Build history of the part. All positions in model axes, mm. Face numbers are marked on the shaded views. A direction names the side the tool comes from. Give positions to 0.01 mm unless a question says otherwise; leave off trailing zeros. Order: outer loops, then holes, each group sorted by start corner. A loop starts at its lowest first (then second) coordinate and runs counter-clockwise, first axis right, second up. Notation, with made-up numbers: (-7, 18.25) -> (50, 18.25) arc R27 ccw to (50, 57.25) -> close; hole circle Ø5 at (54, 2). An arc over 180 degrees is marked (long way). One line per item, written item: value. Start each with the question number.
(1) Saw through at B-B on z = -14.5. Give the cut face in (x, y), plus the area to 3 significant figures.
(2) Pin check, flat tips, straight feed: pin 1 (5 mm diameter, centred on x = 24, z = -0.5, fed in from +Y); pin 2 (1.6 mm diameter, centred on y = 0.5, z = 5, fed in from -X). Stop position of each tip, or through.
(3) Which spindle directions (+Z, -Z, +X, -X, +Y, -Y) get a long thin tool onto all of the face, cutting with end or side? Do the marked faces 5 and 6. Say none if no direction does.
(4) Saw through at A-A on x = -20. Give the cut face in (y, z), plus the area to 3 significant figures.
(5) Saw through at C-C on y = 3.25. Give the cut face in (x, z), plus the area to 3 significant figures.
(6) Probe line 1 (Z direction, x = 10.5, y = 4.5); line 2 (Z direction, x = 14, y = 4.25); line 3 (Z direction, x = -19, y = 6.75). List the from-to ranges inside material, lowest first.
(7) Saw through at D-D on x = -10.5. Give the cut face in (y, z).
(8) Two-plate mould, pull along X, no slides. Class the marked faces 1, 2, 3 and 4: +X half, -X half, draft (parallel to the pull), parting line (faces both ways), or undercut.
Autodesk Inventor part; units mm, degrees
ref_plane "YZ Plane" through (0, 0, 0) normal (1, 0, 0) x (0, 1, 0)
ref_plane "XZ Plane" through (0, 0, 0) normal (0, 1, 0) x (-1, 0, 0)
ref_plane "XY Plane" through (0, 0, 0) normal (0, 0, 1) x (1, 0, 0)
sketch "Sketch1" plane through (0, 0, 0) normal (0, 1, 0) x (-1, 0, 0)
  line L0 (21, 10.5) -> (-21, 10.5)
  line L1 (-21, 10.5) -> (-21, -10.5)
  line L2 (-21, -10.5) -> (21, -10.5)
  line L3 (21, -10.5) -> (21, 10.5)
  line L4 (21, 10.5) -> (-21, -10.5) construction
  line L5 (-21, 10.5) -> (21, -10.5) construction
  line L6 (-29, 18.5) -> (29, 18.5)
  line L7 (29, 18.5) -> (29, -18.5)
  line L8 (29, -18.5) -> (-29, -18.5)
  line L9 (-29, -18.5) -> (-29, 18.5)
  circle A0 centre (10.5, 14.5) radius 1.75
  line L10 (0, 10.5) -> (0, -10.5) construction
  line L11 (-21, 0) -> (21, 0) construction
  circle A1 centre (10.5, -14.5) radius 1.75
  circle A2 centre (-10.5, 14.5) radius 1.75
  circle A3 centre (-10.5, -14.5) radius 1.75
  line L12 (-21, 10.5) -> (-27, 10.5)
  line L13 (-27, 10.5) -> (-27, -10.5)
  line L14 (-27, -10.5) -> (-21, -10.5)
  line L15 (-21, -10.5) -> (-21, 10.5)
  line L16 (21, 10.5) -> (27, 10.5)
  line L17 (27, 10.5) -> (27, -10.5)
  line L18 (27, -10.5) -> (21, -10.5)
  point P0 (0, 0)
  dimension "d0" = 21
  dimension "d1" = 42
  dimension "d2" = 8
  dimension "d3" = 3.5
  dimension "d4" = 10.5
  dimension "d5" = 4
  dimension "d6" = 6
  dimension "d7" = 21
extrude "Extrusion1" add sketch "Sketch1" along normal blind 8
extrude "Extrusion2" add sketch "Sketch1" along normal blind 2 contours L16 L17 L18 L3 | L1 L14 L13 L12
fillet "Fillet1" radius 8 2 edges at (-29, 4, 18.5) (29, 4, 18.5)
fillet "Fillet2" radius 2 4 edges at (-27, 5, 10.5) (-27, 5, -10.5) (27, 5, 10.5) (27, 5, -10.5)
fillet "Fillet3" radius 2 10 edges at (-26.6569, 0, 16.1569) (0, 0, 18.5) (26.6569, 0, 16.1569) (29, 0, -4) (-29, 0, -4) (-26.6569, 8, 16.1569) (0, 8, 18.5) (26.6569, 8, 16.1569) (29, 8, -4) (-29, 8, -4)
equation "\"d0\" = MountWidth"
equation "\"d1\" = MountLength"
equation "\"d2\" = MountThickness"
equation "\"d3\" = THROUGH_DIAMETER"
equation "\"d4\" = 0.25 * MountLength"
equation "\"d5\" = 0.5 * MountThickness"
equation "\"d7\" = MountWidth"
equation "\"d8\" = OUTER_HEIGHT"
equation "\"d12\" = OUTER_FILLET"
equation "\"d13\" = INNER_FILLET"
equation "\"d14\" = PART_FILLET"
properties part number "CoxaServoCutout"
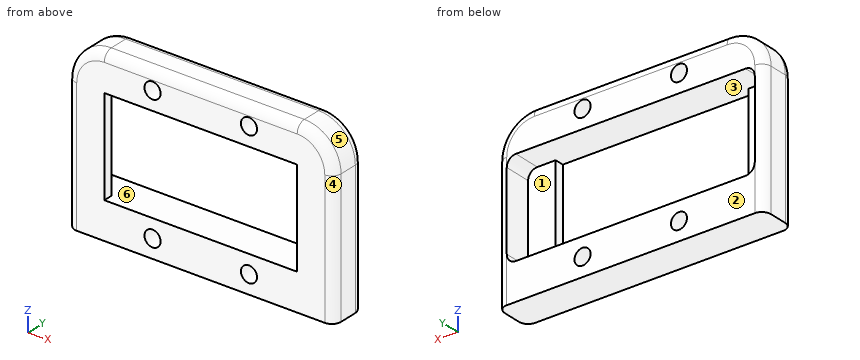
Results below:
1. outline: (-29, 2) arc R2 ccw to (-27, 0) -> (-12.25, 0) -> (-12.25, 8) -> (-27, 8) arc R2 ccw to (-29, 6) -> close; (-8.75, 0) -> (8.75, 0) -> (8.75, 8) -> (-8.75, 8) -> close; (12.25, 0) -> (27, 0) arc R2 ccw to (29, 2) -> (29, 6) arc R2 ccw to (27, 8) -> (12.25, 8) -> close
1. area: 405 mm²
2. pin 1: stops at y = 2
2. pin 2: stops at x = -28.87
3. face 5: +Z, +X, +Y, -Y
3. face 6: +Y
4. outline: (0, -18.5) -> (8, -18.5) -> (8, -10.5) -> (0, -10.5) -> close; (0, 10.5) -> (8, 10.5) -> (8, 16.5) arc R2 ccw to (6, 18.5) -> (2, 18.5) arc R2 ccw to (0, 16.5) -> close
4. area: 126 mm²
5. outline: (-29, -18.5) -> (29, -18.5) -> (29, 10.5) arc R8 ccw to (21, 18.5) -> (-21, 18.5) arc R8 ccw to (-29, 10.5) -> close; hole (-27, -8.5) arc R2 ccw to (-25, -10.5) -> (25, -10.5) arc R2 ccw to (27, -8.5) -> (27, 8.5) arc R2 ccw to (25, 10.5) -> (-25, 10.5) arc R2 ccw to (-27, 8.5) -> close; hole circle Ø3.5 at (-10.5, -14.5); hole circle Ø3.5 at (-10.5, 14.5); hole circle Ø3.5 at (10.5, -14.5); hole circle Ø3.5 at (10.5, 14.5)
5. area: 949 mm²
6. line 1: z = -18.5 to -16.25, -12.75 to -10.5, 10.5 to 12.75, 16.25 to 18.5
6. line 2: z = -18.5 to -10.5, 10.5 to 18.5
6. line 3: z = -18.5 to -10.5, 10.5 to 18.35
7. outline: (0, -18.5) -> (8, -18.5) -> (8, -16.25) -> (0, -16.25) -> close; (0, -12.75) -> (8, -12.75) -> (8, -10.5) -> (0, -10.5) -> close; (0, 10.5) -> (8, 10.5) -> (8, 12.75) -> (0, 12.75) -> close; (0, 16.25) -> (8, 16.25) -> (8, 16.5) arc R2 ccw to (6, 18.5) -> (2, 18.5) arc R2 ccw to (0, 16.5) -> close
8. face 1: undercut
8. face 2: draft
8. face 3: undercut
8. face 4: +X half
